```python
from build123d import *

# Parameters (mm, degrees)
BOSS_EXTRU_1_DEPTH      = 45
ENL_V_MAT_EXTRU_1_DEPTH = 0.5
CONG_1_R                = 0.25
CONG_2_R                = 2
ESQUISSE3_R             = 1.5
ENL_V_MAT_EXTRU_2_DEPTH = 1


with BuildPart() as part:
    # Esquisse1 → Boss.-Extru.1 (new body)
    with BuildSketch(Plane.XY):
        with BuildLine():
            Line((-11.1, 8.5), (11.1, 8.5))
            ThreePointArc((11.1, 8.5), (12.514213562, 7.914213562), (13.1, 6.5))
            Line((13.1, 6.5), (13.1, -6.5))
            ThreePointArc((13.1, -6.5), (12.514213562, -7.914213562), (11.1, -8.5))
            Line((11.1, -8.5), (-11.1, -8.5))
            ThreePointArc((-11.1, -8.5), (-12.514213562, -7.914213562), (-13.1, -6.5))
            Line((-13.1, -6.5), (-13.1, 6.5))
            ThreePointArc((-13.1, 6.5), (-12.514213562, 7.914213562), (-11.1, 8.5))
        make_face()
    extrude(amount=BOSS_EXTRU_1_DEPTH)

    # Esquisse2 → Enlèv. mat.-Extru.1 (cut)
    with BuildSketch(Plane(origin=(0, 0, 0), x_dir=(-1, 0, 0), z_dir=(0, 0, -1))):
        with BuildLine():
            Line((11.6, -6.5), (11.6, 6.5))
            ThreePointArc((11.6, 6.5), (11.453553391, 6.853553391), (11.1, 7))
            Line((11.1, 7), (-11.1, 7))
            ThreePointArc((-11.1, 7), (-11.453553391, 6.853553391), (-11.6, 6.5))
            Line((-11.6, 6.5), (-11.6, -6.5))
            ThreePointArc((-11.6, -6.5), (-11.453553391, -6.853553391), (-11.1, -7))
            Line((-11.1, -7), (11.1, -7))
            ThreePointArc((11.1, -7), (11.453553391, -6.853553391), (11.6, -6.5))
        make_face()
    extrude(amount=-ENL_V_MAT_EXTRU_1_DEPTH, mode=Mode.SUBTRACT)

    # Congé1
    cong_1_edges = [part.edges().sort_by_distance(p)[0] for p in [
        (-13.1, 0, 0),
        (-12.514213562, 7.914213562, 0),
        (-11.453553391, 6.853553391, 0),
        (0, 7, 0),
        (11.453553391, 6.853553391, 0),
        (11.6, 0, 0),
        (11.453553391, -6.853553391, 0),
        (0, -7, 0),
        (-11.453553391, -6.853553391, 0),
        (-11.6, 0, 0),
        (0, 8.5, 0),
        (12.514213562, 7.914213562, 0),
        (13.1, 0, 0),
        (12.514213562, -7.914213562, 0),
        (0, -8.5, 0),
        (-12.514213562, -7.914213562, 0),
    ]]
    fillet(cong_1_edges, radius=CONG_1_R)

    # Congé2
    cong_2_edges = [part.edges().sort_by_distance(p)[0] for p in [
        (-12.514213562, -7.914213562, 45),
        (0, -8.5, 45),
        (12.514213562, -7.914213562, 45),
        (13.1, 0, 45),
        (12.514213562, 7.914213562, 45),
        (0, 8.5, 45),
        (-12.514213562, 7.914213562, 45),
        (-13.1, 0, 45),
    ]]
    fillet(cong_2_edges, radius=CONG_2_R)

    # Esquisse3 → Enlèv. mat.-Extru.2 (cut)
    with BuildSketch(Plane(origin=(0, 0, 0.5), x_dir=(-1, 0, 0), z_dir=(0, 0, -1))):
        with Locations((-6.25, 0)):
            Circle(ESQUISSE3_R)
        with Locations((6.25, 0)):
            Circle(ESQUISSE3_R)
    extrude(amount=-ENL_V_MAT_EXTRU_2_DEPTH, mode=Mode.SUBTRACT)


solid = part.part
```
Build history of the part. All positions in model axes, mm. A direction names the side the tool comes from. Give positions to 0.01 mm unless a question says otherwise; leave off trailing zeros. Order: outer loops, then holes, each group sorted by start corner. A loop starts at its lowest first (then second) coordinate and runs counter-clockwise, first axis right, second up. Notation, with made-up numbers: M 9,-28 L 66,-28 A26 cw 66,-12 Z; hole C 60.25,28 d9. An arc over 180 degrees is marked long. Return JSON: item names as keys, results as strings.
Q1. Two-plate mould, pull along Y, no slides. Class faces 1 (the face through (12.5, 7.93, 21.33)), 2 (the face through (-6, 0, 1.5)), 3 (the face through (13.1, 0, 21)), 4 (the face through (-12.5, -7.93, 21.33)): pulls with the +Y half, pulls with the -Y half, needs draft (parallel to the pull), parting line crosses it, or undercut.
Answer list:
{"face 1": "pulls with the +Y half", "face 2": "undercut", "face 3": "needs draft", "face 4": "pulls with the -Y half"}
Q2. Flat gauge pins, fed straight in: pin 1 (3.5 mm diameter, centred on x = 6.5, y = 0.5, fed in from -Z); pin 2 (0.9 mm diameter, centred on x = -6.5, y = 0.5, fed in from -Z). Where does each tip first touch, or does it go through?
Answer list:
{"pin 1": "stops at z = 0.5", "pin 2": "stops at z = 1.5"}
Q3. 3-axis set-ups, long thin cutter, end or side, ignore diameter. For faces 5 (the face through (12.53, -7.9, 21.33)), 6 (the face through (7.44, -0.91, 0.99)): which of +Z, -Z, +X, -X, +Y, -Y reach the whole face in a straight line?
Answer list:
{"face 5": "+Z, -Z, +X, -Y", "face 6": "-Z"}
Q4. Band-saw the part on B-B (y = 0). Give the cut face in (x, z), then the cut area to 3 significant figures.
Answer list:
{"outline": "M -13.1,0.25 A0.25 ccw -12.85,0 L -11.85,0 A0.25 ccw -11.6,0.25 L -11.6,0.5 L -7.75,0.5 L -7.75,1.5 L -4.75,1.5 L -4.75,0.5 L 4.75,0.5 L 4.75,1.5 L 7.75,1.5 L 7.75,0.5 L 11.6,0.5 L 11.6,0.25 A0.25 ccw 11.85,0 L 12.85,0 A0.25 ccw 13.1,0.25 L 13.1,43 A2 ccw 11.1,45 L -11.1,45 A2 ccw -13.1,43 Z", "area": "1,160 mm^2"}
Q5. Band-saw the part on A-A (x = 6.25). Give the cut face in (y, z).
Answer list:
{"outline": "M -8.5,0.25 A0.25 ccw -8.25,0 L -7.25,0 A0.25 ccw -7,0.25 L -7,0.5 L -1.5,0.5 L -1.5,1.5 L 1.5,1.5 L 1.5,0.5 L 7,0.5 L 7,0.25 A0.25 ccw 7.25,0 L 8.25,0 A0.25 ccw 8.5,0.25 L 8.5,43 A2 ccw 6.5,45 L -6.5,45 A2 ccw -8.5,43 Z"}
Q6. Wall check: probe 1 along Y at (x, z) = (-6.25, 0.7); probe 2 along Z at (x, y) = (-5, -1.5); probe 3 along X at (y, z) = (7, 5). Give the ranges that are in metal, low to high. Write a range as from..to.
Answer list:
{"probe 1": "y = -8.5..-1.5, 1.5..8.5", "probe 2": "z = 0.5..45", "probe 3": "x = -13.04..13.04"}
